```python
from build123d import *

# Parameters (mm, degrees)
F0_R     = 3
F0_R_2   = 6
F1_DEPTH = 12
F3_DEPTH = 5
F4_R     = 2.75
F5_DEPTH = 25
F6_R     = 2.5
F6_R_2   = 2.1
F7_DEPTH = 12
F8_R     = 5
F8_R_2   = 3
F8_R_3   = 2.75
F9_DEPTH = 5.4


with BuildPart() as f1:
    # F0 (on Top) → F1 (new body)
    with BuildSketch(Plane.XY):
        with BuildLine():
            Line((-45, -25), (45, -25))
            Line((45, -25), (45, 15))
            Line((45, 15), (35, 25))
            Line((35, 25), (-45, 25))
            Line((-45, 25), (-45, 13))
            Line((-45, 13), (7, 13))
            ThreePointArc((7, 13), (12.656854, 10.656854), (15, 5))
            Line((15, 5), (15, 1))
            ThreePointArc((15, 1), (12.656854, -4.656854), (7, -7))
            Line((7, -7), (-45, -7))
            Line((-45, -7), (-45, -25))
        make_face()
        with Locations((-32.5, 19)):
            Circle(F0_R, mode=Mode.SUBTRACT)
        with Locations((32, 0)):
            Circle(F0_R_2, mode=Mode.SUBTRACT)
        with Locations((2.5, 19)):
            Circle(F0_R, mode=Mode.SUBTRACT)
        with BuildLine():
            Line((-45, 13), (-45, -7))
            Line((-45, -7), (7, -7))
            ThreePointArc((7, -7), (12.656854, -4.656854), (15, 1))
            Line((15, 1), (15, 5))
            ThreePointArc((15, 5), (12.656854, 10.656854), (7, 13))
            Line((7, 13), (-45, 13))
        make_face()
    extrude(amount=F1_DEPTH)

    # F2 (on face) → F3 (cut)
    with BuildSketch(Plane.XY.offset(12)):
        with BuildLine():
            Line((-45, 13), (-45, -7))
            Line((-45, -7), (7, -7))
            ThreePointArc((7, -7), (12.656854, -4.656854), (15, 1))
            Line((15, 1), (15, 5))
            ThreePointArc((15, 5), (12.656854, 10.656854), (7, 13))
            Line((7, 13), (-45, 13))
        make_face()
    extrude(amount=-F3_DEPTH, mode=Mode.SUBTRACT)

    # F4 (on face) → F5 (cut)
    with BuildSketch(Plane.XY.offset(12)):
        with Locations((-32.5, -13)):
            Circle(F4_R)
        with Locations((2.5, -13)):
            Circle(F4_R)
    extrude(amount=-F5_DEPTH, mode=Mode.SUBTRACT)

    # F6 (on face) → F7 (cut)
    with BuildSketch(Plane.XZ.offset(25)):
        with Locations((-40, 6)):
            Circle(F6_R)
        with Locations((-25, 6)):
            Circle(F6_R_2)
        with Locations((25, 6)):
            Circle(F6_R_2)
        with Locations((40, 6)):
            Circle(F6_R)
    extrude(amount=-F7_DEPTH, mode=Mode.SUBTRACT)

    # F8 (on face) → F9 (cut)
    with BuildSketch(Plane(origin=(0, 0, 0), x_dir=(1, 0, 0), z_dir=(0, 0, -1))):
        with Locations((2.5, -19)):
            Circle(F8_R)
        with Locations((2.5, -19)):
            Circle(F8_R_2, mode=Mode.SUBTRACT)
        with Locations((2.5, 13)):
            Circle(F8_R)
        with Locations((2.5, 13)):
            Circle(F8_R_3, mode=Mode.SUBTRACT)
        with Locations((-32.5, -19)):
            Circle(F8_R)
        with Locations((-32.5, -19)):
            Circle(F8_R_2, mode=Mode.SUBTRACT)
        with Locations((-32.5, 13)):
            Circle(F8_R)
        with Locations((-32.5, 13)):
            Circle(F8_R_3, mode=Mode.SUBTRACT)
    extrude(amount=-F9_DEPTH, mode=Mode.SUBTRACT)


solid = f1.part
```
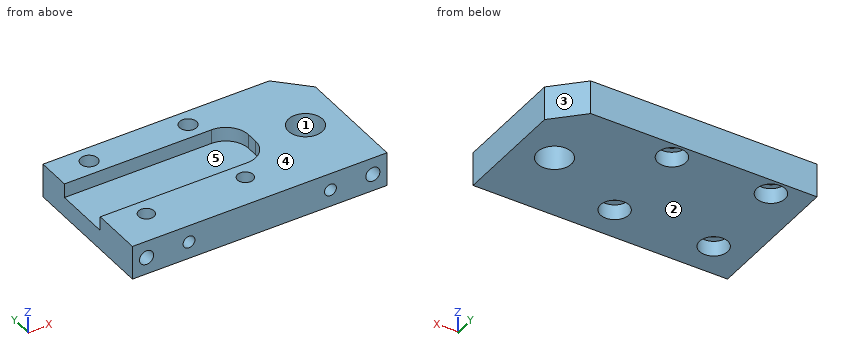
Part model, mm, in its own coordinate system. Face numbers are marked on the shaded views. A direction names the side the tool comes from. Coordinates: 2 decimals unless noted, no trailing zeros. Order: outer loops, then holes, each group sorted by start corner. A loop starts at its lowest first (then second) coordinate and runs counter-clockwise, first axis right, second up. Notation, with made-up numbers: (56, 2) - (74, 2) arc R16 cw to (74, 19) - close; hole circle Ø6 at (24.5, 51.25). An arc over 180 degrees is marked (long way). Return JSON: item names as keys, results as strings. Group by question number.
Item 1: Cut at A-A (x = -32.5). List the corners of the cut face in (y, z), plus the area to 3 significant figures.
Item 2: Drill centre lines: probe 1 along X at (y, z) = (-13, 3.3); probe 2 along Y at (x, z) = (2.5, 8.25); probe 3 along Y at (x, z) = (2.5, 3.95). Where is each one in solid material? Low to high. Write a range as from..to.
Item 3: Cut at B-B (y = -21). List the corners of the cut face in (x, z), plus the area to 3 significant figures.
Item 4: Pull direction X, two halves, no side cores. Call the marked faces 1, 2 and 3: pulls with the +X half, pulls with the -X half, needs draft (parallel to the pull), parting line crosses it, or undercut.
Item 5: Pin check, flat tips, straight feed: pin 1 (1.2 mm diameter, centred on y = 2.5, z = 9.5, fed in from -X); pin 2 (5 mm diameter, centred on x = 4, y = 18, fed in from -Z); pin 3 (4 mm diameter, centred on x = 25, z = 6, fed in from -Y); pin 4 (4.5 mm diameter, centred on x = -32.5, y = -13, fed in from -Z). Stop position of each tip, or through.
Item 6: Which spindle directions (+Z, -Z, +X, -X, +Y, -Y) get a long thin tool onto all of the face, cutting with end or side? Do the marked faces 4 and 5. Say none if no direction does.
Item 7: Cut at D-D (z = 10.5). List the corners of the cut face in (x, y).
Item 8: Cut at C-C (x = 32). List the corners of the cut face in (y, z), plus the area to 3 significant figures.
Check values:
{
 "1": {"outline": "(-25, 0) - (-18, 0) - (-18, 5.4) - (-15.75, 5.4) - (-15.75, 12) - (-25, 12) - close; (-10.25, 5.4) - (-8, 5.4) - (-8, 0) - (14, 0) - (14, 5.4) - (16, 5.4) - (16, 12) - (13, 12) - (13, 7) - (-7, 7) - (-7, 12) - (-10.25, 12) - close; (22, 5.4) - (24, 5.4) - (24, 0) - (25, 0) - (25, 12) - (22, 12) - close", "area": "316 mm2"},
 "2": {"probe 1": "x = -45..-37.5, -27.5..-2.5, 7.5..45", "probe 2": "y = -25..-15.75, -10.25..-7, 13..16, 22..25", "probe 3": "y = -25..-18, -8..14, 24..25"},
 "3": {"outline": "(-45, 0) - (45, 0) - (45, 12) - (-45, 12) - close; hole circle Ø5 at (-40, 6); hole circle Ø4.2 at (-25, 6); hole circle Ø4.2 at (25, 6); hole circle Ø5 at (40, 6)", "area": "1,010 mm2"},
 "4": {"face 1": "undercut", "face 2": "needs draft", "face 3": "pulls with the +X half"},
 "5": {"pin 1": "stops at x = 15", "pin 2": "stops at z = 5.4", "pin 3": "stops at y = -13", "pin 4": "passes through"},
 "6": {"face 4": "+Z, +X, -X, +Y, -Y", "face 5": "+Z, -X"},
 "7": {"outline": "(-45, -25) - (45, -25) - (45, 15) - (35, 25) - (-45, 25) - (-45, 13) - (7, 13) arc R8 cw to (15, 5) - (15, 1) arc R8 cw to (7, -7) - (-45, -7) - close; hole circle Ø6 at (-32.5, 19); hole circle Ø5.5 at (-32.5, -13); hole circle Ø6 at (2.5, 19); hole circle Ø5.5 at (2.5, -13); hole circle Ø12 at (32, 0)"},
 "8": {"outline": "(-25, 0) - (-6, 0) - (-6, 12) - (-25, 12) - close; (6, 0) - (25, 0) - (25, 12) - (6, 12) - close", "area": "456 mm2"}
}
